```python
from build123d import *

# Parameters (mm, degrees)
F0_R     = 4.75
F0_R_2   = 3.6
F1_DEPTH = 10.5
F2_DEPTH = 2
F3_DEPTH = 7.5
F4_W     = 1
F4_H     = 2.5
F5_DEPTH = 1
F6_R     = 0.2
F7_R     = 1


with BuildPart() as f1:
    # F0 (on Front) → F1 (new body)
    with BuildSketch(Plane.XZ):
        Circle(F0_R)
        Circle(F0_R_2, mode=Mode.SUBTRACT)
        Circle(F0_R_2)
        with BuildLine():
            ThreePointArc((-1.8761663039, -1.05), (-0.5425598799, 2.0804155298), (2.15, 0))
            ThreePointArc((2.15, 0), (2.0804155298, -0.5425598799), (1.8761663039, -1.05))
            ThreePointArc((1.8761663039, -1.05), (0, -2.15), (-1.8761663039, -1.05))
        make_face(mode=Mode.SUBTRACT)
        with BuildLine():
            ThreePointArc((1.8761663039, -1.05), (2.0804155298, -0.5425598799), (2.15, 0))
            ThreePointArc((2.15, 0), (-0.5425598799, 2.0804155298), (-1.8761663039, -1.05))
            Line((-1.8761663039, -1.05), (1.8761663039, -1.05))
        make_face()
        with BuildLine():
            Line((1.8761663039, -1.05), (-1.8761663039, -1.05))
            ThreePointArc((-1.8761663039, -1.05), (0, -2.15), (1.8761663039, -1.05))
        make_face()
    extrude(amount=F1_DEPTH)

    # F0 (on Front) → F2 (cut)
    with BuildSketch(Plane.XZ):
        Circle(F0_R_2)
        with BuildLine():
            ThreePointArc((-1.8761663039, -1.05), (-0.5425598799, 2.0804155298), (2.15, 0))
            ThreePointArc((2.15, 0), (2.0804155298, -0.5425598799), (1.8761663039, -1.05))
            ThreePointArc((1.8761663039, -1.05), (0, -2.15), (-1.8761663039, -1.05))
        make_face(mode=Mode.SUBTRACT)
        with BuildLine():
            ThreePointArc((1.8761663039, -1.05), (2.0804155298, -0.5425598799), (2.15, 0))
            ThreePointArc((2.15, 0), (-0.5425598799, 2.0804155298), (-1.8761663039, -1.05))
            Line((-1.8761663039, -1.05), (1.8761663039, -1.05))
        make_face()
        with BuildLine():
            Line((1.8761663039, -1.05), (-1.8761663039, -1.05))
            ThreePointArc((-1.8761663039, -1.05), (0, -2.15), (1.8761663039, -1.05))
        make_face()
    extrude(amount=F2_DEPTH, mode=Mode.SUBTRACT)

    # F0 (on Front) → F3 (cut)
    with BuildSketch(Plane.XZ):
        with BuildLine():
            ThreePointArc((1.8761663039, -1.05), (2.0804155298, -0.5425598799), (2.15, 0))
            ThreePointArc((2.15, 0), (-0.5425598799, 2.0804155298), (-1.8761663039, -1.05))
            Line((-1.8761663039, -1.05), (1.8761663039, -1.05))
        make_face()
    extrude(amount=F3_DEPTH, mode=Mode.SUBTRACT)

    # F4 (on face) → F5 (cut)
    with BuildSketch(Plane.XZ.offset(10.5)):
        with Locations((0, 2.1555542984)):
            Rectangle(F4_W, F4_H)
    extrude(amount=-F5_DEPTH, mode=Mode.SUBTRACT)

    # F6
    f6_edges = [f1.edges().sort_by_distance(p)[0] for p in [
        (-0.5, -10.5, 2.155554),
        (0, -10.5, 3.405554),
        (0.5, -10.5, 2.155554),
        (0, -10.5, 0.905554),
        (0, -9.5, 3.405554),
        (0.5, -9.5, 2.155554),
        (-0.5, -9.5, 2.155554),
        (0, -9.5, 0.905554),
    ]]
    fillet(f6_edges, radius=F6_R)

    # F7
    f7_edges = [f1.edges().sort_by_distance(p)[0] for p in [
        (-4.75, -10.5, 0),
    ]]
    fillet(f7_edges, radius=F7_R)


solid = f1.part
```
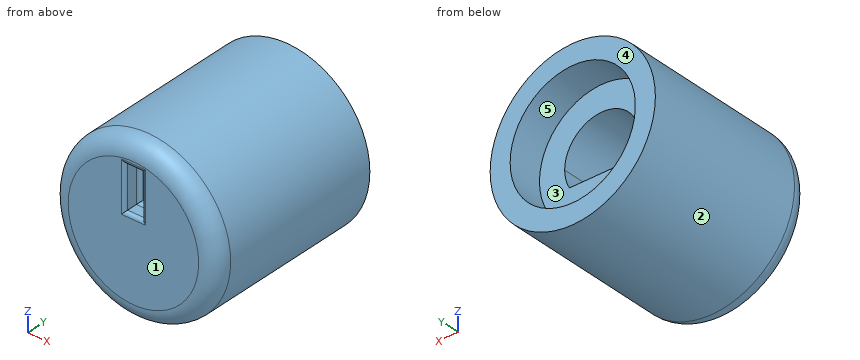
For this review, take the finished solid that the model builds, in its own axes (mm). Face numbers are marked on the shaded views. A direction names the side the tool comes from. Coordinates: 2 decimals unless noted, no trailing zeros. Loops run counter-clockwise (first coordinate to the right, second up) from the corner with the lowest first, then second, coordinate; pieces in that order, holes last.
1. Insertion check: P1, Ø3.5, axis at x = 0.5, z = 0.5, coming from the +Y side; P2, Ø0.7, axis at y = -10, z = 1.5, coming from the -X side; P3, Ø1.5, axis at y = -9.5, z = -1, coming from the +X side. Each pin has a flat end and moves straight along its axis. Give the tip position at first contact, or say it passes through.
2. For the marked faces 4 and 5, list the 3-axis set-ups (+Z, -Z, +X, -X, +Y, -Y) from which the entire face can be reached by the end or side of a thin tool; tool diameter is ignored.
3. Add section B-B, the plane y = -0.5. Give the boundary of the cut face in (x, z), then the cut area to 3 significant figures.
4. Add section C-C, the plane y = -6.5. Give the boundary of the cut face in (x, z), then the cut area to 3 significant figures.
5. Mouldability with a two-part tool opening along Z and no side actions: class the marked faces 1, 2 and 3 as +Z half, -Z half, draft (parallel to the pull), parting line (faces both ways), or undercut.
6. For line 1 (Z direction, x = 0, y = -3.95); line 2 (Z direction, x = 0, y = -1.15); line 3 (Y direction, x = 1.75, z = -2), list the stretches that pass through material, from the lowest coordinate up.
7. Add section A-A, the plane x = 0. Give the boundary of the cut face in (y, z), then the cut area to 3 significant figures.
Result:
1. P1: stops at y = -2
1. P2: stops at x = -4.55
1. P3: stops at x = 4.74
2. face 4: +Z, -Z, +X, -X, +Y
2. face 5: +Y
3. outline: circle Ø9.5 at (0, 0); hole circle Ø7.2 at (0, 0)
3. area: 30.2 mm2
4. outline: circle Ø9.5 at (0, 0); hole (-1.88, -1.05) - (1.88, -1.05) arc R2.15 ccw (long way) to start
4. area: 59.3 mm2
5. face 1: draft
5. face 2: parting line
5. face 3: undercut
6. line 1: z = -4.75 to -1.05, 2.15 to 4.75
6. line 2: z = -4.75 to -3.6, 3.6 to 4.75
6. line 3: y = -10.5 to -2
7. outline: (-10.5, -3.75) arc R1 ccw to (-9.5, -4.75) - (0, -4.75) - (0, -3.6) - (-2, -3.6) - (-2, -1.05) - (-7.5, -1.05) - (-7.5, 2.15) - (-2, 2.15) - (-2, 3.6) - (0, 3.6) - (0, 4.75) - (-9.5, 4.75) arc R1 ccw to (-10.5, 3.75) - (-10.5, 3.61) arc R0.2 ccw to (-10.3, 3.41) - (-9.7, 3.41) arc R0.2 cw to (-9.5, 3.21) - (-9.5, 1.11) arc R0.2 cw to (-9.7, 0.91) - (-10.3, 0.91) arc R0.2 ccw to (-10.5, 0.71) - close
7. area: 64.8 mm2
